from build123d import *

# Parameters (mm, degrees)
SKETCH1_W           = 52.578
SKETCH1_H           = 52.578
EXTRUDE1_DEPTH      = 19.9644
EXTRUDE2_START      = -19.9644
SKETCH2_R           = 2.667
EXTRUDE2_DEPTH      = 5.7658
EXTRUDE4_START      = -19.9644
SKETCH6_R           = 5.75437
EXTRUDE4_DEPTH      = 14.1986
FILLET2_R           = 3.81
SKETCH7_R           = 10.16
BOSS_EXTRUDE1_DEPTH = 101.6


with BuildPart() as part:
    # Sketch1 → Extrude1 (new body)
    with BuildSketch(Plane(origin=(0, 0, 0), x_dir=(1, 0, 0), z_dir=(0, 1, 0))):
        Rectangle(SKETCH1_W, SKETCH1_H)
    extrude(amount=EXTRUDE1_DEPTH)

    # Sketch2 → Extrude2 (cut)
    with BuildSketch(Plane(origin=(0, 19.9644, 0), x_dir=(1, 0, 0), z_dir=(0, 1, 0)).offset(EXTRUDE2_START)):
        with Locations((-17.907, 17.907)):
            Circle(SKETCH2_R)
        with Locations((-17.907, -17.907)):
            Circle(SKETCH2_R)
        with Locations((18.02131475, -17.695628339)):
            Circle(SKETCH2_R)
        with Locations((17.907, 17.907)):
            Circle(SKETCH2_R)
    extrude(amount=EXTRUDE2_DEPTH, mode=Mode.SUBTRACT)

    # Sketch6 → Extrude4 (cut)
    with BuildSketch(Plane.XZ.offset(EXTRUDE4_START)):
        with Locations((-17.907, -17.907)):
            Circle(SKETCH6_R)
        with Locations((-17.907, 17.907)):
            Circle(SKETCH6_R)
        with Locations((17.772836554, 17.95632809)):
            Circle(SKETCH6_R)
        with Locations((17.907, -17.907)):
            Circle(SKETCH6_R)
    extrude(amount=EXTRUDE4_DEPTH, mode=Mode.SUBTRACT)

    # Fillet2
    fillet2_edges = [part.edges().sort_by_distance(p)[0] for p in [
        (-26.289, 9.9822, -26.289),
        (26.289, 9.9822, -26.289),
        (26.289, 9.9822, 26.289),
        (-26.289, 9.9822, 26.289),
    ]]
    fillet(fillet2_edges, radius=FILLET2_R)

    # Sketch7 → Boss-Extrude1 (add)
    with BuildSketch(Plane(origin=(0, 0, 0), x_dir=(1, 0, 0), z_dir=(0, 1, 0))):
        Circle(SKETCH7_R)
    extrude(amount=BOSS_EXTRUDE1_DEPTH)


solid = part.part
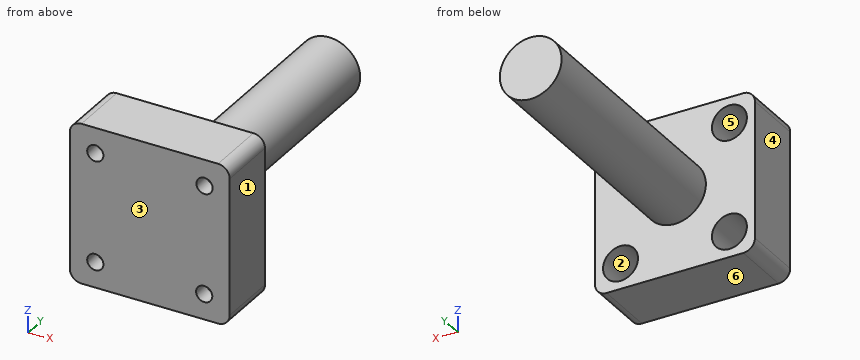
Here's how the part is built. I have some questions about the finished solid (model axes, mm). Face numbers are marked on the shaded views. A direction names the side the tool comes from. Coordinates: 2 decimals unless noted, no trailing zeros. Write each loop counter-clockwise with the first axis right and the second up, starting at its lowest first coordinate (ties: lowest second). Pieces come first, ordered by that corner, then holes.
Item 1: If we mould it in two halves opening along X, with no side actions, what happens to the marked faces 1, 2, 3 and 4? For each: +X half, -X half, draft (parallel to the pull), parting line (faces both ways), or undercut.
Item 2: I want a section at C-C on z = 0. Write out the boundary of the cut face in (x, y).
Item 3: I want a section at D-D on x = 19. Write out the boundary of the cut face in (y, z).
Item 4: I want a section at A-A on x = 0. Write out the boundary of the cut face in (y, z).
Item 5: I want a section at B-B on y = 16. Write out the boundary of the cut face in (x, z), and give its area (3 significant figures).
Item 6: If I drill on line 1 (Y direction, x = 4, z = -13.5); line 2 (Y direction, x = -21.5, z = -21); line 3 (X direction, y = 85.5, z = 1.5), over which ranges is the centre line in solid material (lowest first)?
Item 7: Will these pins go through, and if not, where does the flat tip stop? pin 1 (4 mm diameter, centred on y = 38.5, z = 5.5, fed in from -X); pin 2 (6 mm diameter, centred on x = -15, z = 18.5, fed in from +Y); pin 3 (3.5 mm diameter, centred on x = 20, z = -19, fed in from +Y).
Item 8: On a 3-axis mill with a long thin cutter (end or side, diameter ignored), from which of +Z, -Z, +X, -X, +Y, -Y can I reach the whole of each face in a straight line? I mean the marked faces 5 and 6. Say none if no direction works.
Findings below:
1. face 1: +X half
1. face 2: undercut
1. face 3: draft
1. face 4: -X half
2. outline: (-26.29, 0) - (26.29, 0) - (26.29, 19.96) - (10.16, 19.96) - (10.16, 101.6) - (-10.16, 101.6) - (-10.16, 19.96) - (-26.29, 19.96) - close
3. outline: (0, -26.29) - (19.96, -26.29) - (19.96, -23.56) - (5.77, -23.56) - (5.77, -20.34) - (0, -20.34) - close; (0, -15.47) - (5.77, -15.47) - (5.77, -12.26) - (19.96, -12.26) - (19.96, 12.33) - (5.77, 12.33) - (5.77, 15.21) - (0, 15.21) - close; (0, 20.18) - (5.77, 20.18) - (5.77, 23.58) - (19.96, 23.58) - (19.96, 26.29) - (0, 26.29) - close
4. outline: (0, -26.29) - (19.96, -26.29) - (19.96, -10.16) - (101.6, -10.16) - (101.6, 10.16) - (19.96, 10.16) - (19.96, 26.29) - (0, 26.29) - close
5. outline: (-26.29, -22.48) arc R3.81 ccw to (-22.48, -26.29) - (22.48, -26.29) arc R3.81 ccw to (26.29, -22.48) - (26.29, 22.48) arc R3.81 ccw to (22.48, 26.29) - (-22.48, 26.29) arc R3.81 ccw to (-26.29, 22.48) - close; hole circle Ø11.51 at (-17.91, -17.91); hole circle Ø11.51 at (-17.91, 17.91); hole circle Ø11.51 at (17.77, 17.96); hole circle Ø11.51 at (17.91, -17.91)
5. area: 2,340 mm2
6. line 1: y = 0 to 19.96
6. line 2: y = 0 to 5.77
6. line 3: x = -10.05 to 10.05
7. pin 1: stops at x = -9.54
7. pin 2: stops at y = 19.96
7. pin 3: stops at y = 5.77
8. face 5: +Y
8. face 6: -Z, +X, -X, +Y, -Y
